Input: part model. Units: mm. Frame: model coordinates. A direction names the side the tool comes from. Give positions to 0.01 mm unless a question says otherwise; leave off trailing zeros. Write each loop counter-clockwise with the first axis right and the second up, starting at its lowest first coordinate (ties: lowest second). Pieces come first, ordered by that corner, then holes. Notation, with made-up numbers: (49, -31.75) -> (57, -31.75) arc R16 ccw to (57, -8.75) -> close; hole circle Ø6 at (-28.5, 3.25). An arc over 180 degrees is marked (long way). Return JSON: item names as keys, results as strings. Group by question number.
Item 1: Set-up query: faces 1 (the face through (3.81, 5, -5)), 2 (the face through (0, 6.35, 0)), 3 (the face through (-3.81, 5, 5)). Return all of +Z, -Z, +X, -X, +Y, -Y with unobstructed straight access to the full face (end or side cutting, diameter ignored); none if empty.
Item 2: Section A-A, the plane z = 0. Return loops of the section in (x, y), then the cut area to 3 significant figures.
Item 3: Line query: line 1 (Y direction, x = -2.75, z = -0.5); line 2 (Y direction, x = -2.5, z = -7); line 3 (Z direction, x = 1.75, y = -3). Output: solid intervals per line, ascending. Write a range as [from, to].
Item 4: Pin query (flat end, axial travel): P1, Ø5, axis at x = 0.5, z = 7, coming from the +Y side; P2, Ø3, axis at x = -1.5, y = 6.5, coming from the -Z side; P3, Ø2, axis at x = -3.5, z = -6, coming from the -Y side. Return the tip coordinate at first contact, or that it passes through.
Item 5: Mould query, pull axis Y, two halves, no side actions, for faces 4 (the face through (5.08, -12, -4)), 5 (the face through (0, 17, -4)), 6 (the face through (0.053, -3.219, -5.474)). Classes: released by +Y, released by -Y, zero draft, split by the parting line, or undercut.
from build123d import *

# Parameters (mm, degrees)
CUT_EXTRUDE1_REACH = 28.247


with BuildPart() as part:
    # Sketch2 → Revolve1 (revolve)
    with BuildSketch(Plane.XY, mode=Mode.PRIVATE) as revolve1_sk:
        with BuildLine():
            Line((-5.08, 17.4625), (-5.08, 12.3825))
            ThreePointArc((-5.08, 12.3825), (-4.181974388, 12.010525612), (-3.81, 11.1125))
            Line((-3.81, 11.1125), (-3.81, 0))
            Line((-3.81, 0), (3.81, 0))
            Line((3.81, 0), (3.81, 11.1125))
            ThreePointArc((3.81, 11.1125), (4.181974388, 12.010525612), (5.08, 12.3825))
            Line((5.08, 12.3825), (5.08, 17.4625))
            Line((5.08, 17.4625), (-5.08, 17.4625))
        make_face()
    revolve(revolve1_sk.sketch.rotate(Axis((-6.869429095, 0, 0), (1, 0, 0)), 90), axis=Axis((-6.869429095, 0, 0), (1, 0, 0)))

    # Sketch3 → Cut-Extrude1 (cut, up to next)
    with BuildSketch(Plane(origin=(3.81, 0, 0), x_dir=(0, 0, -1), z_dir=(1, 0, 0)), mode=Mode.PRIVATE) as cut_extrude1_sk1:
        Polygon((7.332348419, 0), (3.666174209, 6.35), (-3.666174209, 6.35), (-7.332348419, 0), (-3.666174209, -6.35), (3.666174209, -6.35), align=None)
    cut_extrude1_tool1 = extrude(cut_extrude1_sk1.sketch, amount=-CUT_EXTRUDE1_REACH, mode=Mode.PRIVATE) & part.part
    add(cut_extrude1_tool1.solids().sort_by_distance((3.81, 0, 0))[0], mode=Mode.SUBTRACT)


solid = part.part
Answer below:
{
 "1": {"face 1": "+X", "face 2": "+X, -X", "face 3": "-X"},
 "2": {"outline": "(-5.08, -17.46) -> (5.08, -17.46) -> (5.08, -12.38) arc R1.27 cw to (3.81, -11.11) -> (3.81, -6.35) -> (-3.81, -6.35) -> (-3.81, -11.11) arc R1.27 cw to (-5.08, -12.38) -> close; (-5.08, 12.38) arc R1.27 cw to (-3.81, 11.11) -> (-3.81, 6.35) -> (3.81, 6.35) -> (3.81, 11.11) arc R1.27 cw to (5.08, 12.38) -> (5.08, 17.46) -> (-5.08, 17.46) -> close", "area": "197 mm2"},
 "3": {"line 1": "y = [-17.46, -6.35], [6.35, 17.46]", "line 2": "y = [-16, -0.58], [0.58, 16]", "line 3": "z = [-17.2, -5.6], [5.6, 17.2]"},
 "4": {"P1": "stops at y = 16.87", "P2": "stops at z = -16.73", "P3": "stops at y = -16.73"},
 "5": {"face 4": "zero draft", "face 5": "split by the parting line", "face 6": "undercut"}
}
